Part model, mm, in its own coordinate system. A direction names the side the tool comes from. Give positions to 0.01 mm unless a question says otherwise; leave off trailing zeros. Order: outer loops, then holes, each group sorted by start corner. A loop starts at its lowest first (then second) coordinate and runs counter-clockwise, first axis right, second up. Notation, with made-up numbers: (-6.75, 55) - (6.25, 55) arc R30 ccw to (6.25, 93) - close; hole circle Ø9 at (72, 5). An arc over 180 degrees is marked (long way). One line per item, written item: value.
```python
from build123d import *

# Parameters (mm, degrees)
PLATE_SKETCH_W      = 95
PLATE_SKETCH_H      = 95
PLATE_EXTRUDE_DEPTH = 10
PLATE_FILLET_R      = 10
POLE_SKETCH_R       = 30
POLE_SKETCH_R_2     = 20
POLE_EXTRUDE_DEPTH  = 700


with BuildPart() as part:
    # Plate Sketch → Plate Extrude (new body)
    with BuildSketch(Plane.XY):
        Rectangle(PLATE_SKETCH_W, PLATE_SKETCH_H)
    extrude(amount=PLATE_EXTRUDE_DEPTH)

    # Plate Fillet
    plate_fillet_edges = [part.edges().sort_by_distance(p)[0] for p in [
        (47.5, -47.5, 5),
        (-47.5, -47.5, 5),
        (-47.5, 47.5, 5),
        (47.5, 47.5, 5),
    ]]
    fillet(plate_fillet_edges, radius=PLATE_FILLET_R)

    # Pole Sketch → Pole Extrude (add)
    with BuildSketch(Plane.XY.offset(10)):
        Circle(POLE_SKETCH_R)
        Circle(POLE_SKETCH_R_2, mode=Mode.SUBTRACT)
    extrude(amount=POLE_EXTRUDE_DEPTH)


solid = part.part
```
1) Which spindle directions (+Z, -Z, +X, -X, +Y, -Y) get a long thin tool onto all of the face, cutting with end or side? Do faces 4 (the flat face through (-1, 1, 0)), 5 (the cylindrical face through (-4.336, -19.524, 355.1)). Say none if no direction does.
Outcome:
face 4: -Z, +X, -X, +Y, -Y
face 5: +Z
2) Mould opens along X. For faces 1 (the flat face through (0, 0, 10)), 2 (the flat face through (6, -20, 710)), 3 (the cylindrical face through (-29.97, 1.32, 355.1)) say: released by +X, released by -X, zero draft, split by the parting line, or undercut.
Outcome:
face 1: undercut
face 2: zero draft
face 3: split by the parting line
3) Drill centre lines: line 1 along X through (y, z) = (-1, 165); line 2 along Y through (x, z) = (0, 447); line 3 along Y through (x, z) = (2, 69). Where is each one in solid material? Low to high. Write a range as from..to.
Outcome:
line 1: x = -29.98..-19.97, 19.97..29.98
line 2: y = -30..-20, 20..30
line 3: y = -29.93..-19.9, 19.9..29.93
4) Cut at A-A, the plane y = 0. Give the cut face in (x, z), then the cut area to 4 significant figures.
Outcome:
outline: (-47.5, 0) - (47.5, 0) - (47.5, 10) - (30, 10) - (30, 710) - (20, 710) - (20, 10) - (-20, 10) - (-20, 710) - (-30, 710) - (-30, 10) - (-47.5, 10) - close
area: 14,950 mm^2
5) Pin check, flat tips, straight feed: pin 1 (5 mm diameter, centred on y = 9, z = 134.5, fed in from +X); pin 2 (5 mm diameter, centred on x = -24.5, y = 36, fed in from +Z); pin 3 (1.5 mm diameter, centred on y = 2.5, z = 261, fed in from +X). Stop position of each tip, or through.
Outcome:
pin 1: stops at x = 29.29
pin 2: stops at z = 10
pin 3: stops at x = 29.95
6) Cut at C-C, the plane z = 258. Give the cut face in (x, y), then the cut area to 3 significant figures.
Outcome:
outline: circle Ø60 at (0, 0); hole circle Ø40 at (0, 0)
area: 1,570 mm^2
